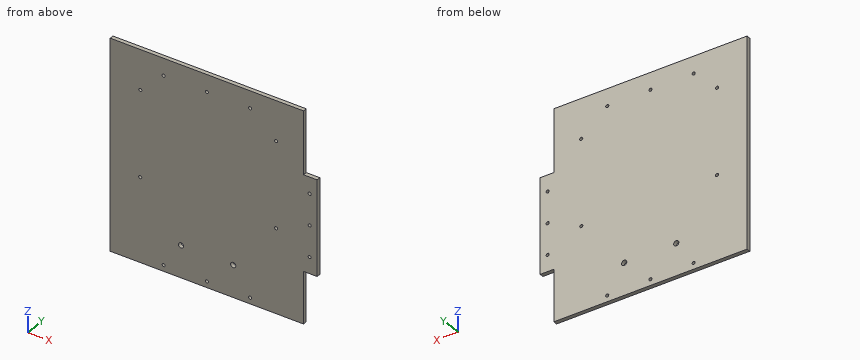
from build123d import *

# Parameters (mm, degrees)
SKETCH1_W           = 313
SKETCH1_H           = 342
BOSS_EXTRUDE1_DEPTH = 6.35
SKETCH3_W           = 22
SKETCH3_H           = 155.14040353
SKETCH3_R           = 2.5
BOSS_EXTRUDE2_DEPTH = 6.35
SKETCH2_R           = 2.5
CUT_EXTRUDE1_DEPTH  = 7.35
SKETCH4_R           = 4.25
SKETCH4_R_2         = 2.5
CUT_EXTRUDE2_DEPTH  = 7.35


with BuildPart() as part:
    # Sketch1 → Boss-Extrude1 (new body)
    with BuildSketch(Plane(origin=(0, 0, 0), x_dir=(1, 0, 0), z_dir=(0, 1, 0))):
        Rectangle(SKETCH1_W, SKETCH1_H)
    extrude(amount=-BOSS_EXTRUDE1_DEPTH)

    # Sketch3 → Boss-Extrude2 (add)
    with BuildSketch(Plane(origin=(0, 0, 0), x_dir=(1, 0, 0), z_dir=(0, 1, 0))):
        with Locations((167.5, 9)):
            Rectangle(SKETCH3_W, SKETCH3_H)
        with Locations((166.5, 9)):
            Circle(SKETCH3_R, mode=Mode.SUBTRACT)
        with Locations((166.5, -41.8)):
            Circle(SKETCH3_R, mode=Mode.SUBTRACT)
        with Locations((166.5, 59.8)):
            Circle(SKETCH3_R, mode=Mode.SUBTRACT)
    extrude(amount=-BOSS_EXTRUDE2_DEPTH)

    # Sketch2 → Cut-Extrude1 (cut, through all)
    with BuildSketch(Plane(origin=(0, 0, 0), x_dir=(1, 0, 0), z_dir=(0, 1, 0))):
        with Locations((0, -143)):
            Circle(SKETCH2_R)
        with Locations((-70, -143)):
            Circle(SKETCH2_R)
        with Locations((70, -143)):
            Circle(SKETCH2_R)
        with Locations((-70, 161)):
            Circle(SKETCH2_R)
        with Locations((0, 161)):
            Circle(SKETCH2_R)
        with Locations((70, 161)):
            Circle(SKETCH2_R)
    extrude(amount=-CUT_EXTRUDE1_DEPTH, mode=Mode.SUBTRACT)

    # Sketch4 → Cut-Extrude2 (cut, through all)
    with BuildSketch(Plane(origin=(0, 0, 0), x_dir=(1, 0, 0), z_dir=(0, 1, 0))):
        with Locations((42.574237453, 118.86741573)):
            Circle(SKETCH4_R)
        with Locations((-41.829962547, 118.86741573)):
            Circle(SKETCH4_R)
        with Locations((-107.911484214, -106.065530058)):
            Circle(SKETCH4_R_2)
        with Locations((-107.911484214, 33.934469942)):
            Circle(SKETCH4_R_2)
        with Locations((112.088515786, 33.934469942)):
            Circle(SKETCH4_R_2)
        with Locations((112.088515786, -106.065530058)):
            Circle(SKETCH4_R_2)
    extrude(amount=-CUT_EXTRUDE2_DEPTH, mode=Mode.SUBTRACT)


solid = part.part
Verification items for the finished model (mm, model axes). Round coordinates to 2 decimals unless told otherwise and drop trailing zeros. Loops run counter-clockwise (first coordinate to the right, second up) from the corner with the lowest first, then second, coordinate; pieces in that order, holes last. Notation, with made-up numbers: (-40, 59.25) - (13, 59.25) arc R24 ccw to (13, 94.25) - close; hole circle Ø3 at (59.25, -0.75). An arc over 180 degrees is marked (long way). Answer in a Markdown table with one row per item. Add a question column.
Q1. Section check B-B on z = 135. Enter the section's corners in (x, y), plus the area to 3 significant figures.
Q2. Material ranges on line 1 (X direction, y = -3, z = 143); line 2 (X direction, y = -3.5, z = 41.8); line 3 (Z direction, x = -107, y = -6), recorded low to high.
Q3. Section check A-A on y = -3.75. State how many separate pieces and enclosed holes the cut face has, plus the area to 3 significant figures.
Q4. Gauge pin test, flat end, axial feed: pin 1 (3 mm diameter, centred on x = 170, y = -3, fed in from +Z). Record the tip position at first contact, or that the pin passes through.
Found:
| question | item | result |
|---|---|---|
| 1 | outline | (-156.5, -6.35) - (156.5, -6.35) - (156.5, 0) - (-156.5, 0) - close |
| 1 | area | 1,990 mm² |
| 2 | line 1 | x = -156.5 to -72.5, -67.5 to -2.5, 2.5 to 67.5, 72.5 to 156.5 |
| 2 | line 2 | x = -156.5 to 164, 169 to 178.5 |
| 2 | line 3 | z = -171 to -36.26, -31.61 to 103.74, 108.39 to 171 |
| 3 | separate pieces | 1 |
| 3 | enclosed holes | 15 |
| 3 | area | 110,000 mm² |
| 4 | pin 1 | stops at z = 68.57 |
